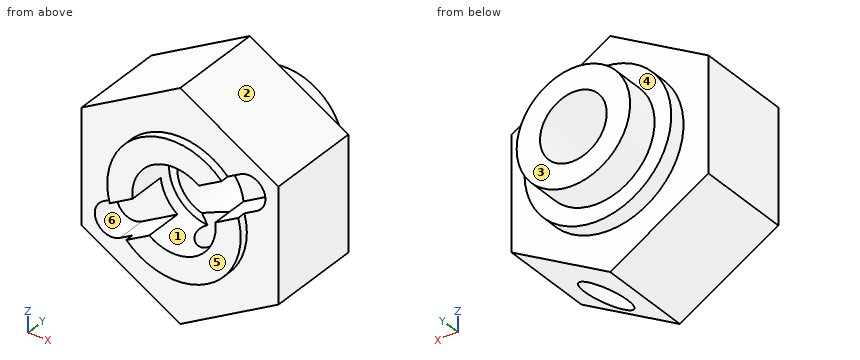
Autodesk Inventor part; units mm, degrees
ref_plane "YZ Plane" through (0, 0, 0) normal (1, 0, 0) x (0, 1, 0)
ref_plane "XZ Plane" through (0, 0, 0) normal (0, 1, 0) x (-1, 0, 0)
ref_plane "XY Plane" through (0, 0, 0) normal (0, 0, 1) x (1, 0, 0)
sketch "Sketch1" plane through (0, 0, 0) normal (0, 1, 0) x (-1, 0, 0)
  line L0 (0, -6.8127) -> (-5.9, -3.4064)
  line L1 (-5.9, -3.4064) -> (-5.9, 3.4064)
  line L2 (-5.9, 3.4064) -> (0, 6.8127)
  line L3 (0, 6.8127) -> (5.9, 3.4064)
  line L4 (5.9, 3.4064) -> (5.9, -3.4064)
  line L5 (5.9, -3.4064) -> (0, -6.8127)
  line L6 (0, -9.5378) -> (0, 9.5378)
  point P0 (0, 0)
  point P1 (0, 0)
  dimension "d0" = 11.8
extrude "Extrusion1" add sketch "Sketch1" along normal blind 5.7
sketch "Sketch2" plane through (0, 5.7, 0) normal (0, 1, 0) x (1, 0, 0)
  circle A0 centre (0, 0) radius 4.4
  dimension "d3" = 8.8
extrude "Extrusion2" add sketch "Sketch2" along normal blind 1
sketch "Sketch3" plane through (0, 6.7, 0) normal (0, 1, 0) x (1, 0, 0)
  circle A0 centre (0, 0) radius 3.4
  dimension "d6" = 6.8
extrude "Extrusion3" add sketch "Sketch3" along normal blind 2
sketch "Sketch4" plane through (0, 0, 0) normal (0, 1, 0) x (-1, 0, 0)
  circle A0 centre (0, 0) radius 4
  dimension "d9" = 8
extrude "Extrusion4" add sketch "Sketch4" against normal blind 0.5
sketch "Sketch5" plane through (0, -0.5, 0) normal (0, -1, 0) x (1, 0, 0)
  circle A0 centre (0, 0) radius 2.5
  dimension "d12" = 5
extrude "Extrusion5" cut sketch "Sketch5" against normal blind 3
sketch "Sketch6" plane through (0, 8.7, 0) normal (0, 1, 0) x (1, 0, 0)
  circle A0 centre (0, 0) radius 2
  dimension "d15" = 4
extrude "Extrusion6" cut sketch "Sketch6" against normal up to next
sketch "Sketch7" plane through (0, -0.5, 0) normal (0, -1, 0) x (1, 0, 0)
  line L0 (-4.1136, -2.375) -> (4.1136, 2.375) construction
  line L1 (-3.6136, -3.241) -> (4.6136, 1.509)
  line L2 (3.6136, 3.241) -> (-4.6136, -1.509)
  arc A0 (-4.6136, -1.509) -> (-3.6136, -3.241) centre (-4.1136, -2.375) ccw
  arc A1 (4.6136, 1.509) -> (3.6136, 3.241) centre (4.1136, 2.375) ccw
  line L3 (0, 6.8127) -> (-5.9, 3.4064)
  point P0 (0, 0)
  point P1 (0, 0)
  dimension "d18" = 11.5
  dimension "d19" = 2
extrude "Extrusion7" cut sketch "Sketch7" against normal blind 2.3
sketch "Sketch8" plane through (0, 0, -6.8127) normal (0.5, 0, -0.8660254) x (-0.8660254, 0, -0.5)
  line L0 (0, 0) -> (0, 5.7) construction
  line L1 (-6.8127, 0) -> (-6.8127, 5.7) construction
  circle A0 centre (-3.4064, 2) radius 1.5
  line L2 (9.6112, 0) -> (-21.9003, 0)
  point P0 (-3.4064, 0)
  dimension "d23" = 3
  dimension "d24" = 2
  dimension "d25" = 0
extrude "Extrusion8" cut sketch "Sketch8" against normal up to surface
thread "Thread1"
properties part number "RCT-H009_tuerca"
Build history of the part. All positions in model axes, mm. Face numbers are marked on the shaded views. A direction names the side the tool comes from. Coordinates: 2 decimals unless noted, no trailing zeros. Order: outer loops, then holes, each group sorted by start corner. A loop starts at its lowest first (then second) coordinate and runs counter-clockwise, first axis right, second up. Notation, with made-up numbers: (0, -36.75) - (12, -36.75) arc R12 ccw to (12, -23.75) - close; hole circle Ø5 at (2, -9). An arc over 180 degrees is marked (long way). Write each question's results on one line, items separated by ' | '. Start each with the question number.
Item 1: Band-saw the part on A-A on y = 4.5. Write the cut outline in (x, z), and give its area (3 significant figures).
Item 2: Band-saw the part on C-C on y = 6.5. Write the cut outline in (x, z).
Item 3: Band-saw the part on B-B on z = 0. Write the cut outline in (x, y), and give its area (3 significant figures).
Item 4: Mould opens along X. For the marked faces 1, 2 and 3 say: released by +X, released by -X, zero draft, split by the parting line, or undercut.
Item 5: Wall check: probe 1 along X at (y, z) = (0.65, 0); probe 2 along X at (y, z) = (5, 0); probe 3 along Z at (x, y) = (0, 7). Give the ranges that are in metal, low to high. Write a range as [from, to].
Item 6: Tool access for the marked faces 4, 5 and 6: list every direction of +Z, -Z, +X, -X, +Y, -Y with a clear straight run to the whole face (end or side of a thin tool).
Item 7: Flat gauge pins, fed straight in: pin 1 (3 mm diameter, centred on x = 0, z = 0, fed in from -Y); pin 2 (2.5 mm diameter, centred on x = -0.5, z = -1, fed in from -Y). Where does each tip first touch, or does it go through?
Numbers:
1) outline: (-5.9, -3.41) - (0, -6.81) - (5.9, -3.41) - (5.9, 3.41) - (0, 6.81) - (-5.9, 3.41) - close; hole circle Ø4 at (0, 0) | area: 108 mm^2
2) outline: circle Ø8.8 at (0, 0); hole circle Ø4 at (0, 0)
3) outline: (-5.9, 0) - (-4, 0) - (-4, -0.5) - (-2.5, -0.5) - (-2.5, 2.5) - (-2, 2.5) - (-2, 8.7) - (-3.4, 8.7) - (-3.4, 6.7) - (-4.4, 6.7) - (-4.4, 5.7) - (-5.9, 5.7) - close; (2, 2.5) - (2.5, 2.5) - (2.5, -0.5) - (4, -0.5) - (4, 0) - (5.9, 0) - (5.9, 5.7) - (4.4, 5.7) - (4.4, 6.7) - (3.4, 6.7) - (3.4, 8.7) - (2, 8.7) - close | area: 53.9 mm^2
4) face 1: undercut | face 2: released by +X | face 3: zero draft
5) probe 1: [-5.9, -2.5], [2.5, 5.9] | probe 2: [-5.9, -2], [2, 5.9] | probe 3: [-3.4, -2], [2, 3.4]
6) face 4: +Y | face 5: +Z, -Z, +X, -X, -Y | face 6: -Y
7) pin 1: through | pin 2: y = 2.5
